Answer from the drawing. Dimensions are ordinates in mm from the lowest x, y and z of the part. Give positions to 0.01 mm unless a question says otherwise; leave off trailing zeros. Order: outer loops, then holes, each group sorted by start corner. A loop starts at its lowest first (then second) coordinate and runs counter-clockwise, first axis right, second up. Notation, with made-up numbers: M -34.5,10.5 L 20.5,10.5 A19 ccw 20.5,40.5 Z; hole C 84.25,38 d1. An arc over 180 degrees is marked long. One line per item, written item: value.
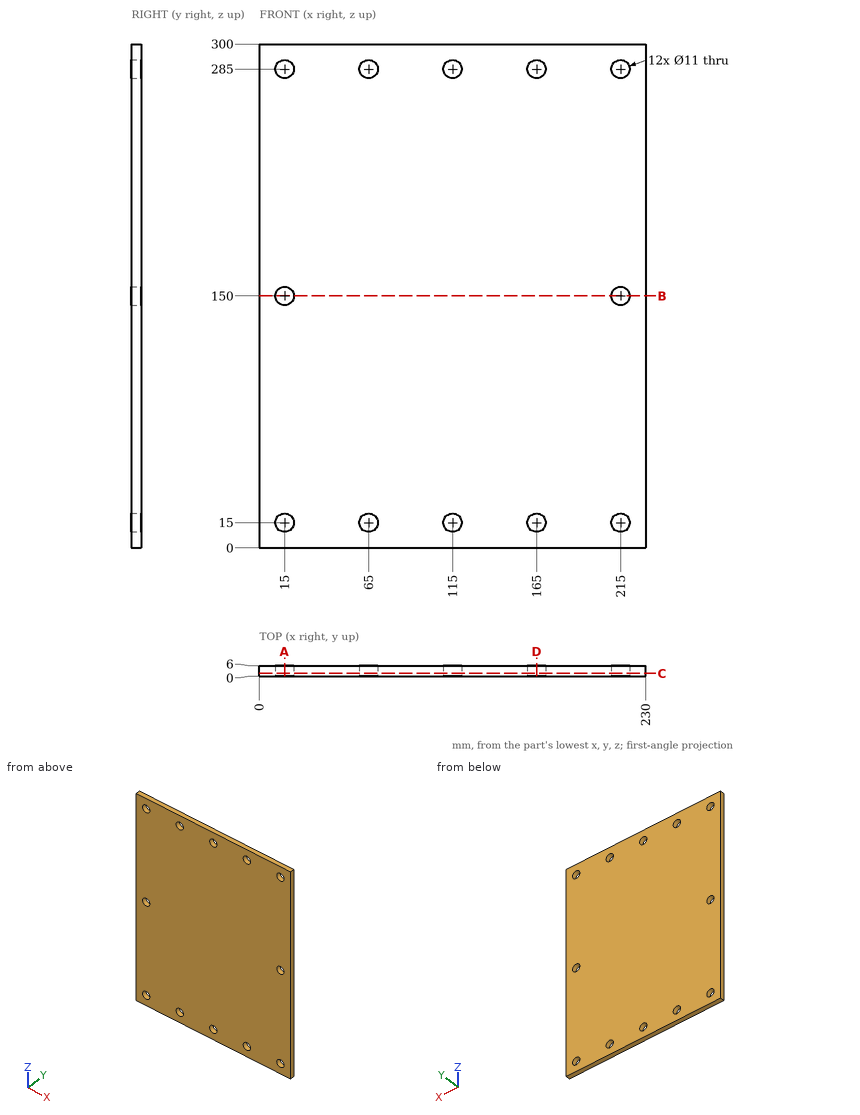
(1) Given P1, Ø10, axis at x = 15, z = 15, coming from the +Y side, flat-ended and moving along its own axis, determine where the tip first touches the part or whether it passes through.
Findings:
P1: passes through
(2) Section C-C, the plane y = 1.55 is taken. Give the number of separate pieces and of enclosed holes in the cut face, then the cut area to 3 significant figures.
Findings:
separate pieces: 1
enclosed holes: 12
area: 67,900 mm^2
(3) Find the intervals of material crossed by probe 1 along X at (y, z) = (4.85, 15); probe 2 along Z at (x, y) = (160.5, 2.3); probe 3 along Z at (x, y) = (212, 1.15), in increasing order. Write a range as from..to.
Findings:
probe 1: x = 0..9.5, 20.5..59.5, 70.5..109.5, 120.5..159.5, 170.5..209.5, 220.5..230
probe 2: z = 0..11.84, 18.16..281.84, 288.16..300
probe 3: z = 0..10.39, 19.61..145.39, 154.61..280.39, 289.61..300
(4) Section B-B, the plane z = 150 is taken. Give the vertices of the cut face in (x, y), then the cut area to 3 significant figures.
Findings:
outline: M 0,0 L 9.5,0 L 9.5,6 L 0,6 Z; M 20.5,0 L 209.5,0 L 209.5,6 L 20.5,6 Z; M 220.5,0 L 230,0 L 230,6 L 220.5,6 Z
area: 1,250 mm^2
(5) Section D-D, the plane x = 165 is taken. Give the vertices of the cut face in (y, z).
Findings:
outline: M 0,0 L 6,0 L 6,9.5 L 0,9.5 Z; M 0,20.5 L 6,20.5 L 6,279.5 L 0,279.5 Z; M 0,290.5 L 6,290.5 L 6,300 L 0,300 Z
(6) Section A-A, the plane x = 15 is taken. Give the vertices of the cut face in (y, z), then the cut area to 3 significant figures.
Findings:
outline: M 0,0 L 6,0 L 6,9.5 L 0,9.5 Z; M 0,20.5 L 6,20.5 L 6,144.5 L 0,144.5 Z; M 0,155.5 L 6,155.5 L 6,279.5 L 0,279.5 Z; M 0,290.5 L 6,290.5 L 6,300 L 0,300 Z
area: 1,600 mm^2
